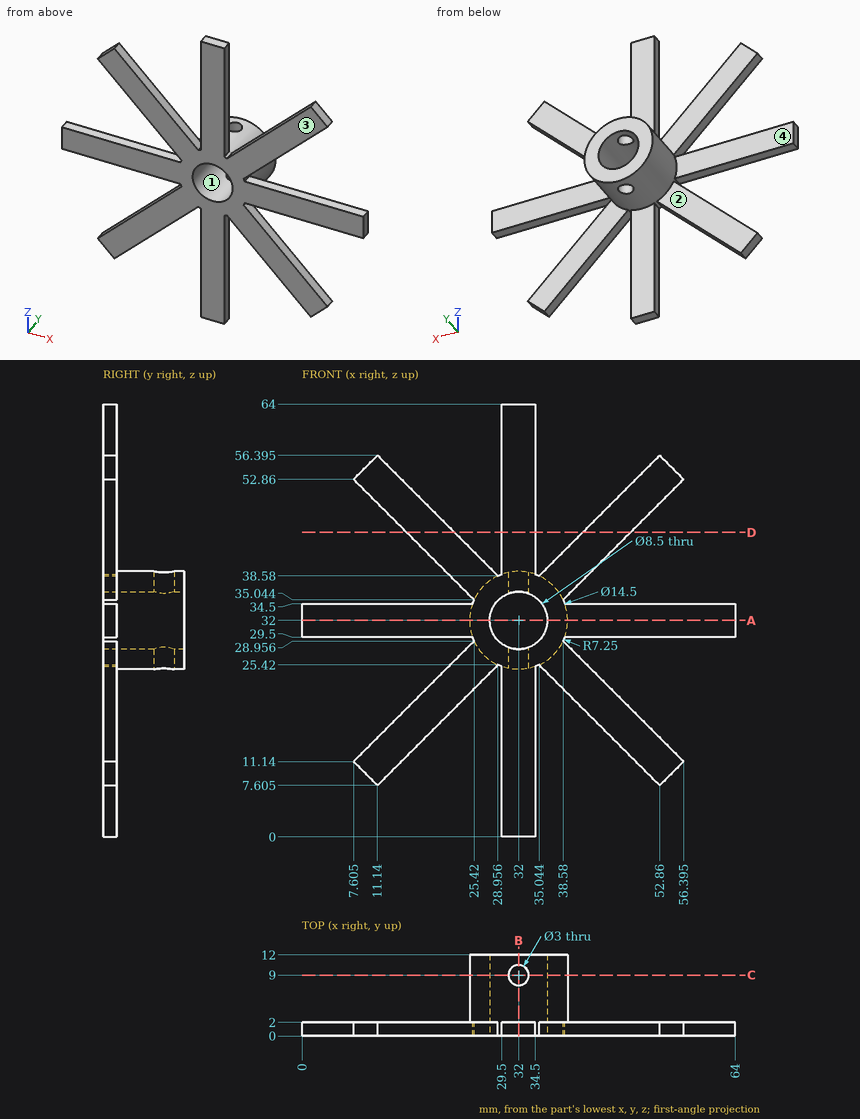
For this review, use the dimensioned drawing (mm, ordinates from the lowest corner) and the shaded views. A direction names the side the tool comes from. Give positions to 0.01 mm unless a question says otherwise; leave off trailing zeros. Loops run counter-clockwise (first coordinate to the right, second up) from the corner with the lowest first, then second, coordinate; pieces in that order, holes last. Notation, with made-up numbers: (15, 80.5) -> (44, 80.5) arc R21 cw to (44, 112.5) -> close; hole circle Ø4 at (46, 74.25). An arc over 180 degrees is marked (long way). One line per question, with ' | ' between items. Start each with the question number.
(1) We need section A-A (z = 32). State the section outline as (x, y) points, and give its area (3 significant figures).
(2) Draft analysis for pull direction Y (two halves, no side actions). For the marked faces 3 and 4, state which applies: +Y half, -Y half, draft (parallel to the pull), parting line (faces both ways), or undercut.
(3) For the marked faces 1 and 2, list the 3-axis set-ups (+Z, -Z, +X, -X, +Y, -Y) from which the entire face can be reached by the end or side of a thin tool; tool diameter is ignored.
(4) For line 1 (Y direction, x = 32, z = 37.85); line 2 (X direction, y = 1, z = 22.5) (1 decimal); line 3 (Z direction, x = 32, y = 6.5), list the stretches that pass through material, from the lowest coordinate up.
(5) We need section B-B (x = 32). State the section outline as (y, z) points, and give its area (3 significant figures).
(6) We need section D-D (z = 45). State the section outline as (x, y) points (1 decimal).
(7) Insertion check: P1, Ø3.5, axis at x = 32, y = 9, coming from the -Z side; P2, Ø2, axis at x = 8.5, y = 0.5, coming from the -Z side (1 decimal); P3, Ø2, axis at x = 36.5, y = 2, coming from the -Z side (1 decimal); P4, Ø3, axis at x = 57, z = 13.5, coming from the -Y side. Each pin has a flat end and moves straight along its axis. Give the tip position at first contact, or say it passes through.
(8) We need section C-C (y = 9). State the section outline as (x, z) points.
The answers:
1) outline: (0, 0) -> (27.75, 0) -> (27.75, 12) -> (24.75, 12) -> (24.75, 2) -> (0, 2) -> close; (36.25, 0) -> (64, 0) -> (64, 2) -> (39.25, 2) -> (39.25, 12) -> (36.25, 12) -> close | area: 171 mm^2
2) face 3: -Y half | face 4: +Y half
3) face 1: +Y, -Y | face 2: -Z, -X, +Y
4) line 1: y = 0 to 7.5, 10.5 to 12 | line 2: x = 19 to 26, 29.5 to 34.5, 38 to 45 | line 3: z = 24.75 to 27.75, 36.25 to 39.25
5) outline: (0, 0) -> (2, 0) -> (2, 24.75) -> (7.5, 24.75) -> (7.5, 27.75) -> (0, 27.75) -> close; (0, 36.25) -> (7.5, 36.25) -> (7.5, 39.25) -> (2, 39.25) -> (2, 64) -> (0, 64) -> close; (10.5, 24.75) -> (12, 24.75) -> (12, 27.75) -> (10.5, 27.75) -> close; (10.5, 36.25) -> (12, 36.25) -> (12, 39.25) -> (10.5, 39.25) -> close | area: 153 mm^2
6) outline: (15.5, 0) -> (22.5, 0) -> (22.5, 2) -> (15.5, 2) -> close; (29.5, 0) -> (34.5, 0) -> (34.5, 2) -> (29.5, 2) -> close; (41.5, 0) -> (48.5, 0) -> (48.5, 2) -> (41.5, 2) -> close
7) P1: stops at z = 24.75 | P2: stops at z = 9.2 | P3: stops at z = 23 | P4: passes through
8) outline: (30.5, 24.91) -> (30.5, 28.02) arc R4.25 cw to (30.5, 35.98) -> (30.5, 39.09) arc R7.25 ccw to start; (33.5, 24.91) arc R7.25 ccw to (33.5, 39.09) -> (33.5, 35.98) arc R4.25 cw to (33.5, 28.02) -> close
